from build123d import *

# Parameters (mm, degrees)
SKETCH1_W                          = 100
SKETCH1_H                          = 100
BOSS_EXTRUDE1_DEPTH                = 2
SKETCH3_W                          = 20.5
SKETCH3_H                          = 20.5
SKETCH3_W_2                        = 4.5
SKETCH3_H_2                        = 4.5
CUT_PEG_HOLE_DEPTH                 = 2
SKETCH4_R                          = 1
CUT_RASPBERRY_PI_SCREW_HOLES_DEPTH = 2
SKETCH5_R                          = 1
CUT_ATHEROS_SCREW_HOLES_DEPTH      = 2


with BuildPart() as part:
    # Sketch1 → Boss-Extrude1 (new body)
    with BuildSketch(Plane(origin=(0, 0, 0), x_dir=(1, 0, 0), z_dir=(0, 1, 0))):
        with Locations((50, 50)):
            Rectangle(SKETCH1_W, SKETCH1_H)
    extrude(amount=BOSS_EXTRUDE1_DEPTH)

    # Sketch3 → Cut - Peg Hole (cut)
    with BuildSketch(Plane(origin=(0, 2, 0), x_dir=(1, 0, 0), z_dir=(0, 1, 0))):
        with Locations((50, 50)):
            Rectangle(SKETCH3_W, SKETCH3_H)
        with Locations((62.5, 50)):
            Rectangle(SKETCH3_W_2, SKETCH3_H_2)
    extrude(amount=-CUT_PEG_HOLE_DEPTH, mode=Mode.SUBTRACT)

    # Sketch4 → Cut - Raspberry Pi Screw Holes (cut)
    with BuildSketch(Plane(origin=(0, 2, 0), x_dir=(1, 0, 0), z_dir=(0, 1, 0))):
        with Locations(Location((4, 26.3, 0), (0, 0, 270))):
            Circle(SKETCH4_R)
        with Locations(Location((4, 4, 0), (0, 0, 270))):
            Circle(SKETCH4_R)
        with Locations(Location((61, 26.3, 0), (0, 0, 270))):
            Circle(SKETCH4_R)
        with Locations(Location((61, 4, 0), (0, 0, 270))):
            Circle(SKETCH4_R)
    extrude(amount=-CUT_RASPBERRY_PI_SCREW_HOLES_DEPTH, mode=Mode.SUBTRACT)

    # Sketch5 → Cut - Atheros Screw Holes (cut)
    with BuildSketch(Plane(origin=(0, 2, 0), x_dir=(1, 0, 0), z_dir=(0, 1, 0))):
        with Locations(Location((3, 67.9, 0), (0, 0, 270))):
            Circle(SKETCH5_R)
        with Locations(Location((14, 67.9, 0), (0, 0, 270))):
            Circle(SKETCH5_R)
        with Locations(Location((14, 97, 0), (0, 0, 270))):
            Circle(SKETCH5_R)
        with Locations(Location((3, 97, 0), (0, 0, 270))):
            Circle(SKETCH5_R)
    extrude(amount=-CUT_ATHEROS_SCREW_HOLES_DEPTH, mode=Mode.SUBTRACT)


solid = part.part
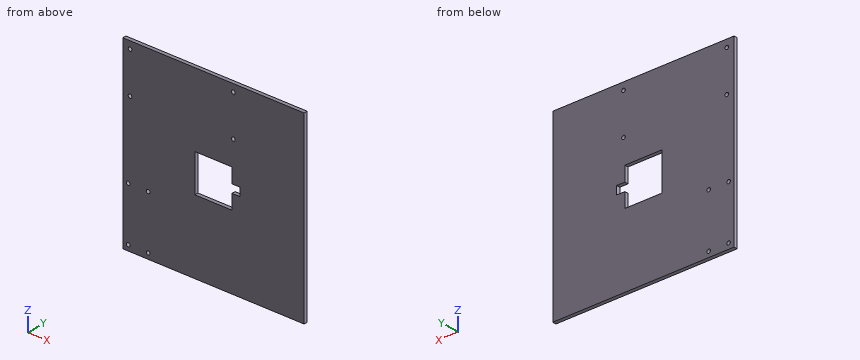
Here's how the part is built. I have some questions about the finished solid (model axes, mm). Coordinates: 2 decimals unless noted, no trailing zeros.
1. For P1, Ø1, axis at x = 59, y = 1, coming from the +Z side, with a flat end and sliding along its axis, tell me the tip position at first contact or that it passes through.
2. I need wall thicknesses on L1, parallel to X at y = 0.85, z = -4; L2, parallel to X at y = 1.5, z = -67.9; L3, parallel to Z at x = 14.5, y = 0.9. Which ranges of each line are inside material? Lowest first, please.
3. Imagine slicing it at A-A, the plane y = 1. Count the separate pieces of the cut face and the enclosed holes in it, and give its area (3 significant figures).
Taken from the geometry:
1. P1: stops at z = 0
2. L1: x = 0 to 3, 5 to 60, 62 to 100
2. L2: x = 0 to 2, 4 to 13, 15 to 100
2. L3: z = -100 to -97.87, -96.13 to -68.77, -67.03 to 0
3. separate pieces: 1
3. enclosed holes: 9
3. area: 9,530 mm2
